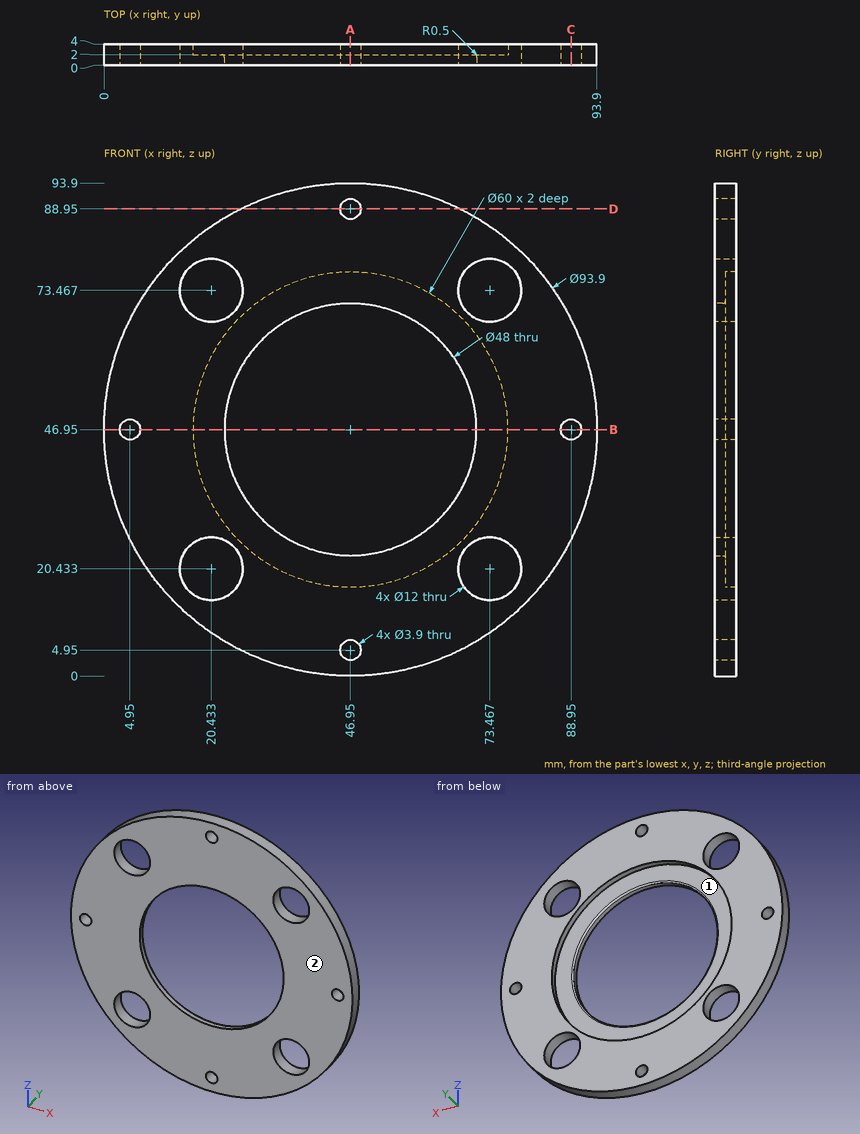
Job drawing, mm, ordinate dimensions from the low corner. One solid piece. Give positions to 0.01 mm unless a question says otherwise; leave off trailing zeros. Loops run counter-clockwise (first coordinate to the right, second up) from the corner with the lowest first, then second, coordinate; pieces in that order, holes last. Notation, with made-up numbers: (10.25, 14) - (35.25, 14) arc R14 ccw to (35.25, 40) - close; hole circle Ø2 at (-11, 58). An arc over 180 degrees is marked (long way). Use one line per item in the form item = value.
(1) Cut at A-A (x = 46.95). Give the cut face in (y, z), then the cut area to 3 significant figures.
Determined:
outline = (0, 0) - (4, 0) - (4, 3) - (0, 3) - close; (0, 6.9) - (4, 6.9) - (4, 16.95) - (2, 16.95) - (2, 22.45) arc R0.5 ccw to (1.5, 22.95) - (0, 22.95) - close; (0, 70.95) - (1.5, 70.95) arc R0.5 ccw to (2, 71.45) - (2, 76.95) - (4, 76.95) - (4, 87) - (0, 87) - close; (0, 90.9) - (4, 90.9) - (4, 93.9) - (0, 93.9) - close
area = 128 mm^2
(2) Cut at B-B (z = 46.95). Give the cut face in (x, y).
Determined:
outline = (0, 0) - (3, 0) - (3, 4) - (0, 4) - close; (6.9, 0) - (22.95, 0) - (22.95, 1.5) arc R0.5 ccw to (22.45, 2) - (16.95, 2) - (16.95, 4) - (6.9, 4) - close; (70.95, 0) - (87, 0) - (87, 4) - (76.95, 4) - (76.95, 2) - (71.45, 2) arc R0.5 ccw to (70.95, 1.5) - close; (90.9, 0) - (93.9, 0) - (93.9, 4) - (90.9, 4) - close
(3) Drop flat-ended pins along their axis: P1, Ø3, axis at x = 46.95, z = 4.95, coming from the +Y side; P2, Ø8, axis at x = 71.5, z = 43, coming from the +Y side; P3, Ø5, axis at x = 4.95, z = 46.95, coming from the -Y side; P4, Ø1.5, axis at y = 1, z = 71, coming from the +X side. Give the stop position or say it passes through.
Determined:
P1 = through
P2 = 2
P3 = 0
P4 = 87.71
(4) Pull direction X, two halves, no side cores. Call the marked faces 1 and 2: pulls with the +X half, pulls with the -X half, needs draft (parallel to the pull), parting line crosses it, or undercut.
Determined:
face_1 = undercut
face_2 = needs draft
(5) Cut at C-C (x = 88.95). Give the cut face in (y, z).
Determined:
outline = (0, 25.97) - (4, 25.97) - (4, 45) - (0, 45) - close; (0, 48.9) - (4, 48.9) - (4, 67.93) - (0, 67.93) - close
(6) Cut at D-D (z = 88.95). Give the cut face in (x, y), then the cut area to 3 significant figures.
Determined:
outline = (25.97, 0) - (45, 0) - (45, 4) - (25.97, 4) - close; (48.9, 0) - (67.93, 0) - (67.93, 4) - (48.9, 4) - close
area = 152 mm^2
(7) Drill centre lines: L1, parallel to X at y = 3.2, z = 46.95; L2, parallel to X at y = 1.3, z = 46.95; L3, parallel to X at y = 1.25, z = 74 (1 decimal). Where is each one in solid material? Low to high.
Determined:
L1 = 0 to 3, 6.9 to 16.95, 76.95 to 87, 90.9 to 93.9
L2 = 0 to 3, 6.9 to 22.95, 70.95 to 87, 90.9 to 93.9
L3 = 8.6 to 14.5, 26.4 to 67.5, 79.4 to 85.3
